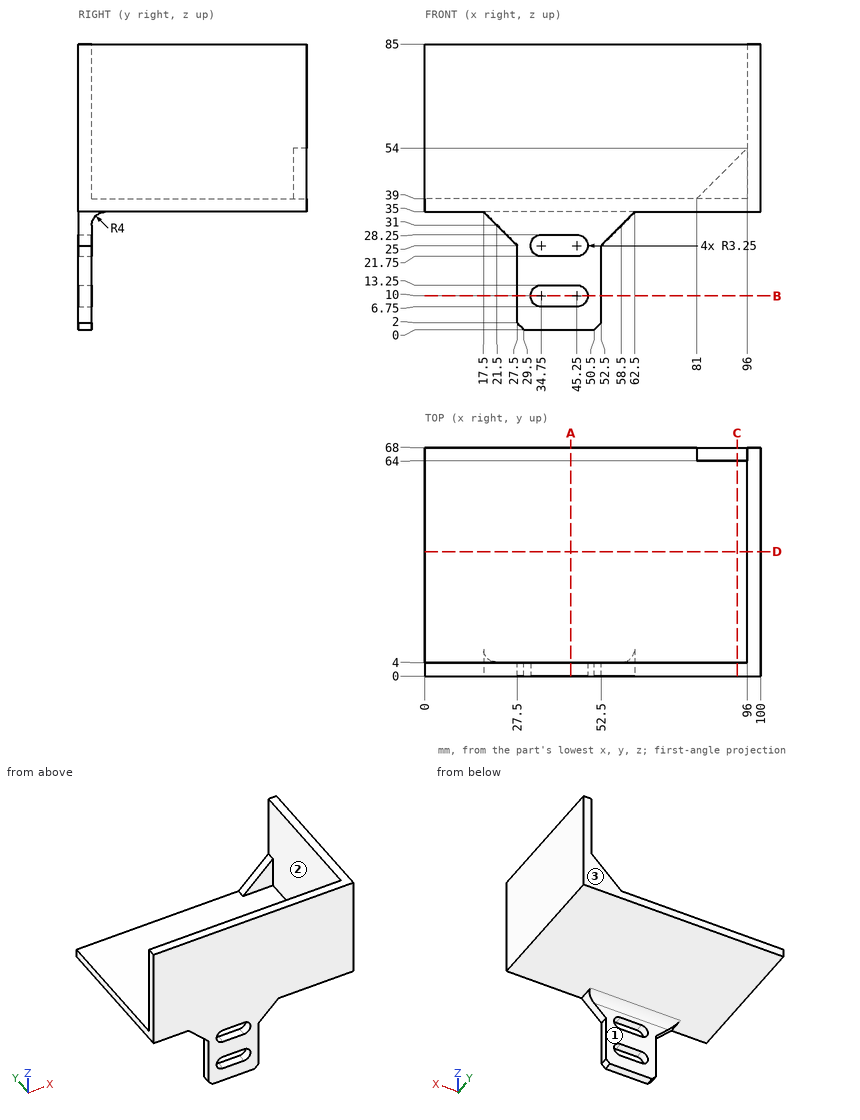
Geometry check sheet. Reference: drawing and pictorial views, mm from the part's lowest x, y, z. A direction names the side the tool comes from. Give positions to 0.01 mm unless a question says otherwise; leave off trailing zeros. Loops run counter-clockwise (first coordinate to the right, second up) from the corner with the lowest first, then second, coordinate; pieces in that order, holes last. Notation, with made-up numbers: (77.5, -19) -> (134.5, -19) arc R12 cw to (134.5, -7) -> close; hole circle Ø9 at (57.5, 6). An arc over 180 degrees is marked (long way). Answer in a Markdown table with one row per item. Add a question column.
1) Set-up check for the marked faces 1, 2 and 3: record each of +Z, -Z, +X, -X, +Y, -Y from which the full face is reachable in a straight line by a thin tool's end or side.
2) Cross-section at A-A on x = 43.5. Record the boundary of the cut face in (y, z), and give its area (3 significant figures).
3) Cross-section at B-B on z = 10. Record the boundary of the cut face in (x, y), and give its area (3 significant figures).
4) Cross-section at D-D on y = 37. Record the boundary of the cut face in (x, z).
5) Cross-section at C-C on x = 93. Record the boundary of the cut face in (y, z).
6) Gauge pin test, flat ends, axial feed: P1, Ø12, axis at x = 19.5, y = 49.5, coming from the -Z side; P2, Ø1.2, axis at y = 2.5, z = 15, coming from the +X side; P3, Ø23, axis at y = 23.5, z = 70.5, coming from the -X side. Record the tip position at first contact, or that the pin passes through.
7) Material ranges on probe 1 along Z at (x, y) = (30, 20); probe 2 along Y at (x, z) = (47.5, 72.5); probe 3 along X at (y, z) = (30, 74), recorded low to high. Write a range as from..to.
Outcome:
| question | item | result |
|---|---|---|
| 1 | face 1 | -Z, +X, -X, +Y |
| 1 | face 2 | +Z, -X |
| 1 | face 3 | +Z, -Z, +X, -X, +Y |
| 2 | outline | (0, 0) -> (4, 0) -> (4, 6.75) -> (0, 6.75) -> close; (0, 13.25) -> (4, 13.25) -> (4, 21.75) -> (0, 21.75) -> close; (0, 28.25) -> (4, 28.25) -> (4, 31) arc R4 cw to (8, 35) -> (68, 35) -> (68, 39) -> (4, 39) -> (4, 85) -> (0, 85) -> close |
| 2 | area | 547 mm^2 |
| 3 | outline | (27.5, 0) -> (31.5, 0) -> (31.5, 4) -> (27.5, 4) -> close; (48.5, 0) -> (52.5, 0) -> (52.5, 4) -> (48.5, 4) -> close |
| 3 | area | 32.0 mm^2 |
| 4 | outline | (0, 35) -> (100, 35) -> (100, 85) -> (96, 85) -> (96, 39) -> (0, 39) -> close |
| 5 | outline | (0, 35) -> (68, 35) -> (68, 51) -> (64, 51) -> (64, 39) -> (4, 39) -> (4, 85) -> (0, 85) -> close |
| 6 | P1 | stops at z = 35 |
| 6 | P2 | stops at x = 52.5 |
| 6 | P3 | stops at x = 96 |
| 7 | probe 1 | z = 35..39 |
| 7 | probe 2 | y = 0..4 |
| 7 | probe 3 | x = 96..100 |
